Read the model definition and answer for the solid it produces. Units are mm, in the model's axes. A direction names the side the tool comes from. Give positions to 0.01 mm unless a question says otherwise; leave off trailing zeros. Order: outer loops, then holes, each group sorted by start corner. A loop starts at its lowest first (then second) coordinate and runs counter-clockwise, first axis right, second up. Notation, with made-up numbers: (16.5, -26.5) - (22.5, -26.5) arc R12 ccw to (22.5, -3.5) - close; hole circle Ø5 at (-1.5, 83). An arc over 180 degrees is marked (long way). Return JSON: item names as keys, results as strings.
```python
from build123d import *

# Parameters (mm, degrees)
SKETCH1_W           = 44.45
SKETCH1_H           = 21.59
BOSS_EXTRUDE1_DEPTH = 12.7
SKETCH2_W           = 7.62
SKETCH2_H           = 19.05
CUT_EXTRUDE1_DEPTH  = 12.7
FILLET1_R           = 1.27
FILLET2_R           = 1.27
SKETCH4_R           = 1.651
CUT_EXTRUDE3_DEPTH  = 12.7
SKETCH5_R           = 1.8034
CUT_EXTRUDE4_DEPTH  = 12.7
SKETCH6_R           = 3.2639
CUT_EXTRUDE5_DEPTH  = 5.08


with BuildPart() as part:
    # Sketch1 → Boss-Extrude1 (new body)
    with BuildSketch(Plane.XY):
        Rectangle(SKETCH1_W, SKETCH1_H)
    extrude(amount=BOSS_EXTRUDE1_DEPTH)

    # Sketch2 → Cut-Extrude1 (cut)
    with BuildSketch(Plane.XY.offset(12.7)):
        with Locations((-18.415, 1.27)):
            Rectangle(SKETCH2_W, SKETCH2_H)
        with Locations((18.415, 1.27)):
            Rectangle(SKETCH2_W, SKETCH2_H)
    extrude(amount=-CUT_EXTRUDE1_DEPTH, mode=Mode.SUBTRACT)

    # Fillet1
    fillet1_edges = [part.edges().sort_by_distance(p)[0] for p in [
        (-14.605, -8.255, 6.35),
    ]]
    fillet(fillet1_edges, radius=FILLET1_R)

    # Fillet2
    fillet2_edges = [part.edges().sort_by_distance(p)[0] for p in [
        (14.605, -8.255, 6.35),
    ]]
    fillet(fillet2_edges, radius=FILLET2_R)

    # Sketch4 → Cut-Extrude3 (cut)
    with BuildSketch(Plane(origin=(0, -8.255, 0), x_dir=(1, 0, 0), z_dir=(0, 1, 0))):
        with Locations(Location((19.05, -6.35, 0), (0, 0, 180))):
            Circle(SKETCH4_R)
        with Locations(Location((-19.05, -6.4262, 0), (0, 0, 180))):
            Circle(SKETCH4_R)
    extrude(amount=-CUT_EXTRUDE3_DEPTH, mode=Mode.SUBTRACT)

    # Sketch5 → Cut-Extrude4 (cut)
    with BuildSketch(Plane(origin=(0, 0, 0), x_dir=(-1, 0, 0), z_dir=(0, 0, -1))):
        with Locations((0, 4.445)):
            Circle(SKETCH5_R)
    extrude(amount=-CUT_EXTRUDE4_DEPTH, mode=Mode.SUBTRACT)

    # Sketch6 → Cut-Extrude5 (cut)
    with BuildSketch(Plane.XY.offset(12.7)):
        with Locations((0, 4.445)):
            Circle(SKETCH6_R)
    extrude(amount=-CUT_EXTRUDE5_DEPTH, mode=Mode.SUBTRACT)


solid = part.part
```
Q1. A cutting plane is placed at A-A (x = 0). Write down the section's boundary in (y, z) (3 decimals).
Values:
{"outline": "(-10.795, 0) - (2.642, 0) - (2.642, 7.62) - (1.181, 7.62) - (1.181, 12.7) - (-10.795, 12.7) - close; (6.248, 0) - (10.795, 0) - (10.795, 12.7) - (7.709, 12.7) - (7.709, 7.62) - (6.248, 7.62) - close"}
Q2. A cutting plane is placed at B-B (x = -19.05). Write down the section's boundary in (y, z) (3 decimals).
Values:
{"outline": "(-10.795, 0) - (-8.255, 0) - (-8.255, 4.775) - (-10.795, 4.775) - close; (-10.795, 8.077) - (-8.255, 8.077) - (-8.255, 12.7) - (-10.795, 12.7) - close"}
Q3. A cutting plane is placed at D-D (y = 1.75). Write down the section's boundary in (x, z) (3 decimals), and give its area (3 significant figures).
Values:
{"outline": "(-14.605, 0) - (14.605, 0) - (14.605, 12.7) - (1.841, 12.7) - (1.841, 7.62) - (-1.841, 7.62) - (-1.841, 12.7) - (-14.605, 12.7) - close", "area": "352 mm²"}
Q4. Determine the mould class of faces 4 (the flat face through (-22.225, -10, 6)), 5 (the flat face through (0, 0, 12.7)), 6 (the cylindrical face through (20.267, -9.507, 7.466)) for opening direction Z: released by +Z, released by -Z, zero draft, split by the parting line, or undercut.
Values:
{"face 4": "zero draft", "face 5": "released by +Z", "face 6": "undercut"}
Q5. Given pin 1 (2 mm diameter, centred on x = 0, y = 4.445, fed in from -Z); pin 2 (1.9 mm diameter, centred on x = -18.5, z = 5, fed in from +Y) (3 decimals); pin 3 (4 mm diameter, centred on y = 6, z = 4, fed in from +X) (3 decimals); pin 4 (7 mm diameter, centred on x = 0, y = 5.5, fed in from +Z), each flat-ended and moving along its own axis, determine where each tip first touches the part or whether it passes through.
Values:
{"pin 1": "passes through", "pin 2": "stops at y = -8.255", "pin 3": "stops at x = 14.605", "pin 4": "stops at z = 12.7"}
Q6. For faces 1 (the flat face through (-17.7, -8.255, 5)), 2 (the cylindrical face through (-0.71, 1.26, 10.2)), 3 (the flat face through (18, -8.255, 8)), determine the directions among +Z, -Z, +X, -X, +Y, -Y from which every point of the face is accessible in a straight line to the end or side of a thin tool.
Values:
{"face 1": "+Z, -Z, -X, +Y", "face 2": "+Z", "face 3": "+Z, -Z, +X, +Y"}
Q7. A cutting plane is placed at C-C (z = 8.75). Write down the section's boundary in (x, y) (3 decimals).
Values:
{"outline": "(-22.225, -10.795) - (22.225, -10.795) - (22.225, -8.255) - (15.875, -8.255) arc R1.27 cw to (14.605, -6.985) - (14.605, 10.795) - (-14.605, 10.795) - (-14.605, -6.985) arc R1.27 cw to (-15.875, -8.255) - (-22.225, -8.255) - close; hole circle Ø6.528 at (0, 4.445)"}
Q8. Consider L1, parallel to Z at x = -19.05, y = -9.3; L2, parallel to Y at x = 0, z = 5.25 (3 decimals); L3, parallel to Z at x = 19.05, y = -9.6. Determine where each line is inside the solid, lowest interval first.
Values:
{"L1": "z = 0 to 4.78, 8.08 to 12.7", "L2": "y = -10.795 to 2.642, 6.248 to 10.795", "L3": "z = 0 to 4.7, 8 to 12.7"}
